Here's how the part is built. I have some questions about the finished solid (model axes, mm). A direction names the side the tool comes from. Coordinates: 2 decimals unless noted, no trailing zeros. Loops run counter-clockwise (first coordinate to the right, second up) from the corner with the lowest first, then second, coordinate; pieces in that order, holes last. Notation, with made-up numbers: M -27.5,25.5 L 0.5,25.5 A30 ccw 0.5,64.5 Z; hole C -1.75,56.25 d9. An arc over 180 degrees is marked long. Use one line per item in the form item = value. Start each with the question number.
(1) Imagine slicing it at B-B, the plane z = 0. Please give me the cut outline in (x, y) (3 decimals), and give its area (3 significant figures).
(2) Will this pin go through, and if not, where does the flat tip stop? P1, Ø0.8, axis at y = -62.5, z = 0, coming from the -X side (3 decimals).
(3) Thinking about a two-plate mould opening in Y: for faces 1 (the flat face through (0, -65, -3.175)), 2 (the flat face through (-12.7, -38, 0)), 3 (the flat face through (0, 0, 0)), 4 (the cylindrical face through (-0.1, -32.43, 8)), which applies, +Y half, -Y half, draft (parallel to the pull), parting line (faces both ways), or undercut?
(4) On a 3-axis mill with a long thin cutter (end or side, diameter ignored), from which of +Z, -Z, +X, -X, +Y, -Y can I reach the whole of each face in a straight line? I mean faces 5 (the cylindrical face through (8.004, -37.367, -0.304)), 6 (the cylindrical face through (-8.004, -61.437, 0.035)), 7 (the cylindrical face through (-0.172, -64.015, -8.004)), 8 (the flat face through (0, -33, 3.175)), 9 (the flat face through (0, -38, 12.7)). Say none if no direction works.
(5) Please list where these lines run through material, in increasing order: L1, parallel to Z at x = 8.5, y = -38.1; L2, parallel to Y at x = 0, z = -8; L3, parallel to Y at x = 0, z = 10.25.
(6) Imagine slicing it at A-A, the plane x = 0. Please give me the cut outline in (y, z) (3 decimals).
(7) Imagine slicing it at C-C, the plane y = -38.1. Please give me the cut outline in (x, z) (3 decimals), and give its area (3 significant figures).
```python
from build123d import *

# Parameters (mm, degrees)
F0_W     = 25.4
F0_H     = 25.4
F1_DEPTH = 76.2
F2_R     = 0.79375
F3_DEPTH = 9.525
F4_R     = 0.79375
F5_DEPTH = 9.525
F6_R     = 0.79375
F7_DEPTH = 9.525
F8_R     = 0.79375
F9_DEPTH = 9.525


with BuildPart() as f1:
    # F0 (on Front) → F1 (new body)
    with BuildSketch(Plane.XZ):
        Rectangle(F0_W, F0_H)
    extrude(amount=F1_DEPTH)

    # F2 (on face) → F3 (cut)
    with BuildSketch(Plane.XY.offset(12.7)):
        with Locations((0, -33.217845)):
            Circle(F2_R)
    extrude(amount=-F3_DEPTH, mode=Mode.SUBTRACT)

    # F4 (on face) → F5 (cut)
    with BuildSketch(Plane.YZ.offset(12.7)):
        with Locations((-38.1, 0)):
            Circle(F4_R)
    extrude(amount=-F5_DEPTH, mode=Mode.SUBTRACT)

    # F6 (on face) → F7 (cut)
    with BuildSketch(Plane(origin=(0, 0, -12.7), x_dir=(1, 0, 0), z_dir=(0, 0, -1))):
        with Locations((0, 64.789804)):
            Circle(F6_R)
    extrude(amount=-F7_DEPTH, mode=Mode.SUBTRACT)

    # F8 (on face) → F9 (cut)
    with BuildSketch(Plane(origin=(-12.7, 0, 0), x_dir=(0, -1, 0), z_dir=(-1, 0, 0))):
        with Locations((62.230002, 0)):
            Circle(F8_R)
    extrude(amount=-F9_DEPTH, mode=Mode.SUBTRACT)


solid = f1.part
```
Answer:
q1.outline = M -12.7,-76.2 L 12.7,-76.2 L 12.7,-38.894 L 3.175,-38.894 L 3.175,-37.306 L 12.7,-37.306 L 12.7,0 L -12.7,0 L -12.7,-61.436 L -3.175,-61.436 L -3.175,-63.024 L -12.7,-63.024 Z
q1.area = 1,910 mm²
q2.P1 = -3.175
q3.face_1 = undercut
q3.face_2 = draft
q3.face_3 = +Y half
q3.face_4 = undercut
q4.face_5 = +X
q4.face_6 = -X
q4.face_7 = -Z
q4.face_8 = +Z
q4.face_9 = +Z, +X, -X, +Y, -Y
q5.L1 = -12.7 to -0.79, 0.79 to 12.7
q5.L2 = -76.2 to -65.58, -64 to 0
q5.L3 = -76.2 to -34.01, -32.42 to 0
q6.outline = M -76.2,-12.7 L -65.584,-12.7 L -65.584,-3.175 L -63.996,-3.175 L -63.996,-12.7 L 0,-12.7 L 0,12.7 L -32.424,12.7 L -32.424,3.175 L -34.012,3.175 L -34.012,12.7 L -76.2,12.7 Z
q7.outline = M -12.7,-12.7 L 12.7,-12.7 L 12.7,-0.794 L 3.175,-0.794 L 3.175,0.794 L 12.7,0.794 L 12.7,12.7 L -12.7,12.7 Z
q7.area = 630 mm²
